Answer from the drawing. Dimensions are ordinates in mm from the lowest x, y and z of the part. Round coordinates to 2 decimals unless told otherwise and drop trailing zeros. Write each loop counter-clockwise with the first axis right and the second up, starting at its lowest first coordinate (ties: lowest second). Pieces come first, ordered by that corner, then holes. Notation, with made-up numbers: (3.25, 29) - (49.25, 29) arc R25 ccw to (49.25, 41) - close; hole circle Ø1 at (67.25, 30.5). An arc over 180 degrees is marked (long way). Return JSON: item names as keys, results as strings. Group by question number.
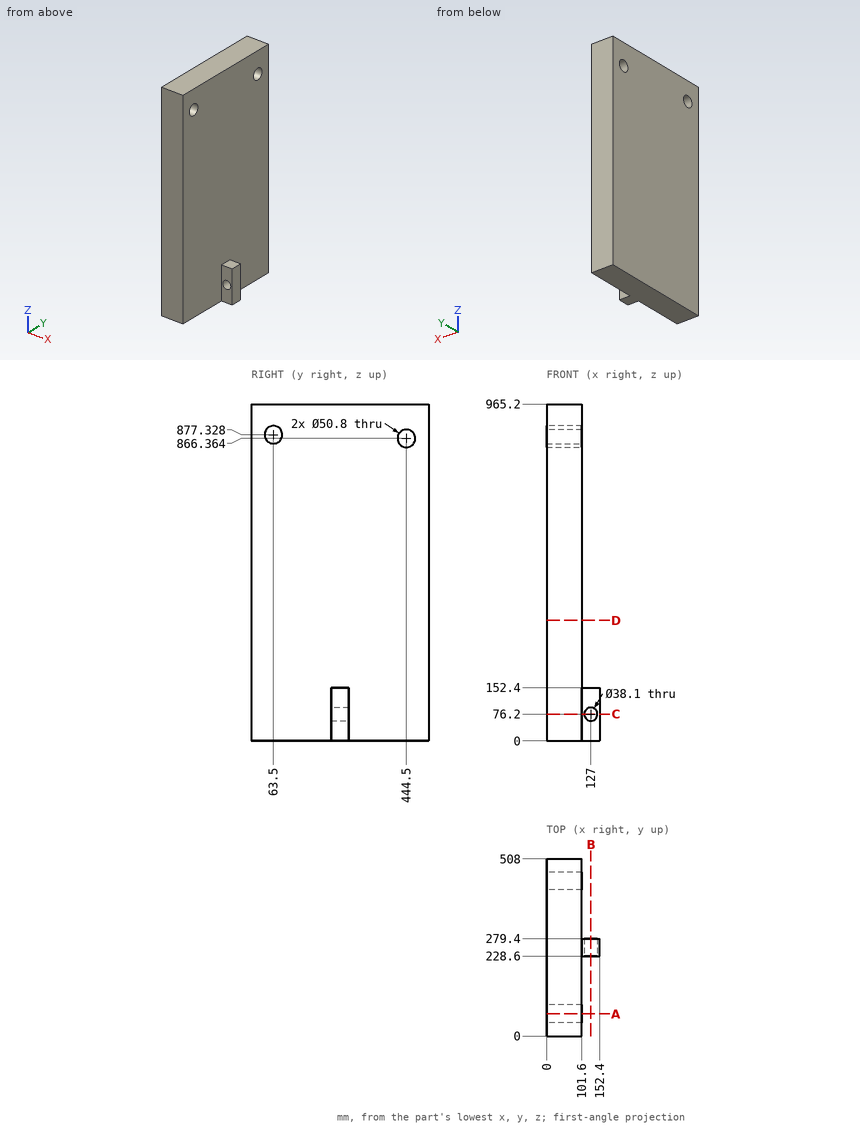
(1) Find section C-C (z = 76.2). Write down the section's boundary in (x, y).
(2) Find section D-D (z = 345). Write down the section's boundary in (x, y).
(3) Find section A-A (y = 63.5). Write down the section's boundary in (x, z), plus the area to 3 significant figures.
(4) A flat-ended cylindrical pin translates along its axis: pin 1 (1 mm diameter, centred on y = 378, z = 348, fed in from +X). Find the tip coordinate at first contact, or state that the pin passes through.
(5) Consider line 1 (Z direction, x = 21, y = 444); line 2 (X direction, y = 245, z = 76.2); line 3 (X direction, y = 60, z = 270). Determine where each line is inside the solid, lowest interval first.
(6) Find section B-B (x = 127). Write down the section's boundary in (y, z), plus the area to 3 significant figures.
Check sheet entries:
{
 "1": {"outline": "(0, 0) - (101.6, 0) - (101.6, 228.6) - (107.95, 228.6) - (107.95, 279.4) - (101.6, 279.4) - (101.6, 508) - (0, 508) - close; (146.05, 228.6) - (152.4, 228.6) - (152.4, 279.4) - (146.05, 279.4) - close"},
 "2": {"outline": "(0, 0) - (101.6, 0) - (101.6, 508) - (0, 508) - close"},
 "3": {"outline": "(0, 0) - (101.6, 0) - (101.6, 851.93) - (0, 851.93) - close; (0, 902.73) - (101.6, 902.73) - (101.6, 965.2) - (0, 965.2) - close", "area": "92,900 mm^2"},
 "4": {"pin 1": "stops at x = 101.6"},
 "5": {"line 1": "z = 0 to 840.97, 891.76 to 965.2", "line 2": "x = 0 to 107.95, 146.05 to 152.4", "line 3": "x = 0 to 101.6"},
 "6": {"outline": "(228.6, 0) - (279.4, 0) - (279.4, 57.15) - (228.6, 57.15) - close; (228.6, 95.25) - (279.4, 95.25) - (279.4, 152.4) - (228.6, 152.4) - close", "area": "5,810 mm^2"}
}
